Input: part model. Units: mm. Frame: model coordinates. Round coordinates to 2 decimals unless told otherwise and drop trailing zeros. Loops run counter-clockwise (first coordinate to the right, second up) from the corner with the lowest first, then second, coordinate; pieces in that order, holes last. Notation, with made-up numbers: M 69.5,5 L 97.5,5 A17 cw 97.5,28 Z; hole C -26.5,40.25 d1. An arc over 180 degrees is marked long. Return JSON: item names as keys, results as strings. Group by question number.
1) Section C-C (z = -9.5). Output: boundary loops of the cut face in (x, y) (3 decimals), plus the area to 3 significant figures.
2) Contact query for flat-ended pins moving along their axis: P1, Ø2.5, axis at x = 69, y = -6.5, coming from the +Z side; P2, Ø0.6, axis at y = -14, z = 3, coming from the +X side; P3, Ø10, axis at x = 32, y = -10, coming from the -Z side. Output: stop coordinate, or through.
3) Material intervals for line 1 (Z direction, x = 11, y = -15); line 2 (X direction, y = -3.25, z = 1.5); line 3 (X direction, y = -14.75, z = -11) (3 decimals), sorted ascending. Write a range as from..to.
4) Section A-A (y = -5.75). Output: boundary loops of the cut face in (x, z) (3 decimals).
5) Section B-B (x = 71.5). Output: boundary loops of the cut face in (y, z) (3 decimals), plus the area to 3 significant figures.
6) Section D-D (x = 17). Output: boundary loops of the cut face in (y, z), plus the area to 3 significant figures.
from build123d import *

# Parameters (mm, degrees)
F1_DEPTH = 19.05


with BuildPart() as f1:
    # F0 (on Front) → F1 (new body)
    with BuildSketch(Plane.XZ):
        with BuildLine():
            Line((3.433455, 0.8128), (11.938, 0.8128))
            ThreePointArc((11.938, 0.8128), (12.476815, 1.035985), (12.7, 1.5748))
            Line((12.7, 1.5748), (12.7, 3.6068))
            ThreePointArc((12.7, 3.6068), (12.476815, 4.145615), (11.938, 4.3688))
            Line((11.938, 4.3688), (-1.905, 4.3688))
            ThreePointArc((-1.905, 4.3688), (-4.150064, 3.438864), (-5.08, 1.1938))
            Line((-5.08, 1.1938), (-5.08, -1.905))
            ThreePointArc((-5.08, -1.905), (-4.150064, -4.150064), (-1.905, -5.08))
            Line((-1.905, -5.08), (70.554239, -5.08))
            Line((70.554239, -5.08), (72.38552, -4.58931))
            ThreePointArc((72.38552, -4.58931), (72.826251, -4.676977), (73.025, -5.08))
            Line((73.025, -5.08), (73.025, -11.43))
            ThreePointArc((73.025, -11.43), (72.826251, -11.833023), (72.38552, -11.92069))
            Line((72.38552, -11.92069), (70.554239, -11.43))
            Line((70.554239, -11.43), (67.437, -11.43))
            ThreePointArc((67.437, -11.43), (66.898185, -11.653185), (66.675, -12.192))
            Line((66.675, -12.192), (66.675, -13.843))
            ThreePointArc((66.675, -13.843), (66.898185, -14.381815), (67.437, -14.605))
            Line((67.437, -14.605), (73.025, -14.605))
            ThreePointArc((73.025, -14.605), (75.270064, -13.675064), (76.2, -11.43))
            Line((76.2, -11.43), (76.2, -3.175))
            ThreePointArc((76.2, -3.175), (75.270064, -0.929936), (73.025, 0))
            Line((73.025, 0), (3.433455, 0))
            Line((3.433455, 0), (0.596213, -0.500282))
            ThreePointArc((0.596213, -0.500282), (0.181464, -0.389151), (0, 0))
            Line((0, 0), (0, 0.8128))
            ThreePointArc((0, 0.8128), (0.181464, 1.201951), (0.596213, 1.313082))
            Line((0.596213, 1.313082), (3.433455, 0.8128))
        make_face()
    extrude(amount=F1_DEPTH)


solid = f1.part
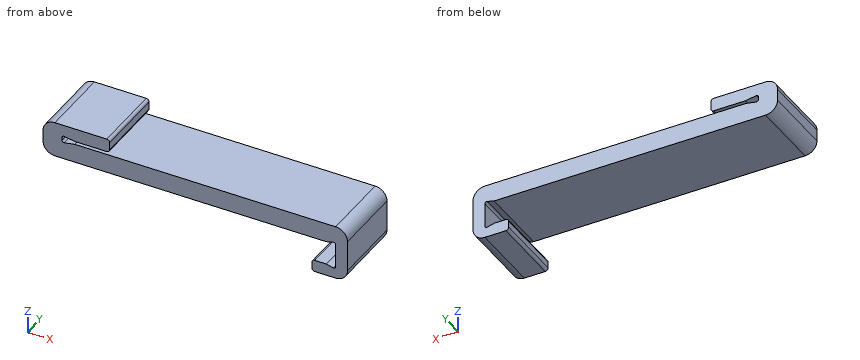
Returned:
{
 "1": {"outline": "M 73.025,-19.05 L 76.2,-19.05 L 76.2,0 L 73.025,0 Z", "area": "60.5 mm^2"},
 "2": {"P1": "stops at z = 0", "P2": "stops at x = 12.7", "P3": "stops at z = -5.08"},
 "3": {"line 1": "z = -5.08..0, 0.81..4.37", "line 2": "x = -5.07..12.7", "line 3": "x = 73.025..76.2"},
 "4": {"outline": "M -5.08,-1.905 A3.175 ccw -1.905,-5.08 L 70.554,-5.08 L 72.386,-4.589 A0.508 cw 73.025,-5.08 L 73.025,-11.43 A0.508 cw 72.386,-11.921 L 70.554,-11.43 L 67.437,-11.43 A0.762 ccw 66.675,-12.192 L 66.675,-13.843 A0.762 ccw 67.437,-14.605 L 73.025,-14.605 A3.175 ccw 76.2,-11.43 L 76.2,-3.175 A3.175 ccw 73.025,0 L 3.433,0 L 0.596,-0.5 A0.508 cw 0,0 L 0,0.813 A0.508 cw 0.596,1.313 L 3.433,0.813 L 11.938,0.813 A0.762 ccw 12.7,1.575 L 12.7,3.607 A0.762 ccw 11.938,4.369 L -1.905,4.369 A3.175 ccw -5.08,1.194 Z"},
 "5": {"outline": "M -19.05,-14.605 L 0,-14.605 L 0,-11.683 L -19.05,-11.683 Z; M -19.05,-4.827 L 0,-4.827 L 0,0 L -19.05,0 Z", "area": "148 mm^2"},
 "6": {"outline": "M -19.05,-5.08 L 0,-5.08 L 0,0 L -19.05,0 Z", "area": "96.8 mm^2"}
}
